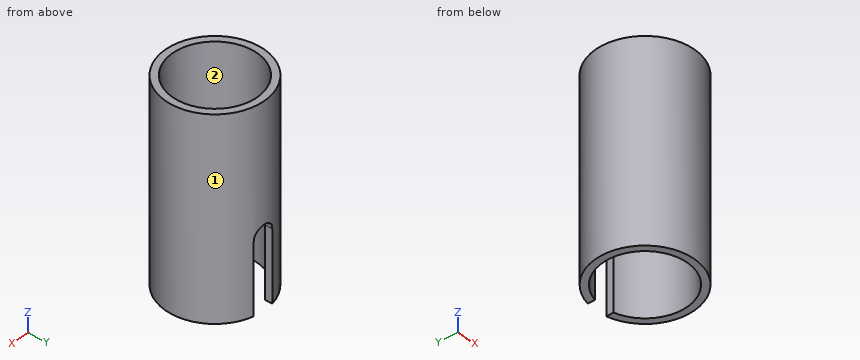
```python
from build123d import *

# Parameters (mm, degrees)
ESQUISSE1_R             = 7
ESQUISSE1_R_2           = 6
BOSS_EXTRU_1_DEPTH      = 14
ENL_V_MAT_EXTRU_1_DEPTH = 18.146428199


with BuildPart() as part:
    # Esquisse1 → Boss.-Extru.1 (new, symmetric)
    with BuildSketch(Plane.XY):
        Circle(ESQUISSE1_R)
        Circle(ESQUISSE1_R_2, mode=Mode.SUBTRACT)
    extrude(amount=BOSS_EXTRU_1_DEPTH, both=True)

    # Esquisse2 → Enlèv. mat.-Extru.1 (cut, through all)
    with BuildSketch(Plane(origin=(0, 0, 0), x_dir=(1, 0, 0), z_dir=(0, 1, 0))):
        with BuildLine():
            Line((-1.5, 82.523499554), (-1.5, 14))
            Line((-1.5, 14), (-1.5, 4))
            ThreePointArc((-1.5, 4), (0, 2.5), (1.5, 4))
            Line((1.5, 4), (1.5, 14))
            Line((1.5, 14), (1.5, 82.523499554))
            Line((1.5, 82.523499554), (1.5, 219.570498661))
            Line((1.5, 219.570498661), (-1.5, 219.570498661))
            Line((-1.5, 219.570498661), (-1.5, 82.523499554))
        make_face()
    extrude(amount=ENL_V_MAT_EXTRU_1_DEPTH, mode=Mode.SUBTRACT)


solid = part.part
```
Can you work these out from the model? Positions are in its coordinate system, mm. Face numbers are marked on the shaded views. Coordinates: 2 decimals unless noted, no trailing zeros. Order: outer loops, then holes, each group sorted by start corner. A loop starts at its lowest first (then second) coordinate and runs counter-clockwise, first axis right, second up.
1. I'm going to push flat-ended pins straight in: pin 1 (4 mm diameter, centred on y = 2.5, z = 6.5, fed in from -X); pin 2 (1.1 mm diameter, centred on y = 6.5, z = -11, fed in from +X); pin 3 (8 mm diameter, centred on x = -2.5, z = -10.5, fed in from +Y). Where does each tip first touch, or does it pass through?
2. Thinking about a two-plate mould opening in Y: for the marked faces 1 and 2, which applies, +Y half, -Y half, draft (parallel to the pull), parting line (faces both ways), or undercut?
3. If we section it at C-C (z = 10.5): Please give me the cut outline in (x, y).
4. If we section it at B-B (x = 0): Please give me the cut outline in (y, z).
5. I need wall thicknesses on line 1 (X direction, y = 0, z = -2); line 2 (X direction, y = -1.25, z = -9.25); line 3 (Y direction, x = 0, z = -2.75). Which ranges of each line are inside material? Lowest first, please.
6. If we section it at A-A (y = 0): Please give me the cut outline in (x, z), then the cut area to 3 significant figures.
7. If we section it at D-D (z = -9.25): Please give me the cut outline in (x, y), then the cut area to 3 significant figures.
Entries:
1. pin 1: stops at x = -6.98
1. pin 2: stops at x = 3.69
1. pin 3: stops at y = 6.84
2. face 1: parting line
2. face 2: undercut
3. outline: circle Ø14 at (0, 0); hole circle Ø12 at (0, 0)
4. outline: (-7, -14) - (-6, -14) - (-6, 14) - (-7, 14) - close; (6, -2.5) - (7, -2.5) - (7, 14) - (6, 14) - close
5. line 1: x = -7 to -6, 6 to 7
5. line 2: x = -6.89 to -5.87, 5.87 to 6.89
5. line 3: y = -7 to -6
6. outline: (-7, -14) - (-6, -14) - (-6, 14) - (-7, 14) - close; (6, -14) - (7, -14) - (7, 14) - (6, 14) - close
6. area: 56.0 mm2
7. outline: (-1.5, 5.81) - (-1.5, 6.84) arc R7 ccw (long way) to (1.5, 6.84) - (1.5, 5.81) arc R6 cw (long way) to start
7. area: 37.8 mm2
